Job drawing, mm, ordinate dimensions from the low corner. One solid piece. A direction names the side the tool comes from. Round coordinates to 2 decimals unless told otherwise and drop trailing zeros. Write each loop counter-clockwise with the first axis right and the second up, starting at its lowest first coordinate (ties: lowest second). Pieces come first, ordered by that corner, then holes.
1) Pull direction Z, two halves, no side cores. Call the marked faces 5, 6, 7 and 8: +Z half, -Z half, draft (parallel to the pull), parting line (faces both ways), or undercut.
2) Saw through at B-B on y = 34.5. Write the cut outline in (x, z), and give its area (3 significant figures).
3) Flat gauge pins, fed straight in: pin 1 (10 mm diameter, centred on x = 7, z = 17.5, fed in from -Y); pin 2 (3.5 mm diameter, centred on y = 23.5, z = 23.5, fed in from +X); pin 3 (0.6 mm diameter, centred on x = 30.5, y = 11, fed in from +Z); pin 4 (2.5 mm diameter, centred on x = 15, z = 15, fed in from +Y). Where does each tip first touch, or does it go through?
4) Saw through at D-D on y = 20.5. Write the cut outline in (x, z).
5) Which spindle directions (+Z, -Z, +X, -X, +Y, -Y) get a long thin tool onto all of the face, cutting with end or side? Do the marked faces 1, 2, 3 and 4. Say none if no direction does.
6) Drill centre lines: L1, parallel to Y at x = 27.5, z = 15; L2, parallel to Z at x = 4, y = 31; L3, parallel to X at y = 36, z = 6.5. Where is each one in solid material? Low to high.
7) Saw through at A-A on z = 15. Write the cut outline in (x, y), and give its area (3 significant figures).
8) Saw through at C-C on x = 15. Write the cut outline in (y, z), and give its area (3 significant figures).
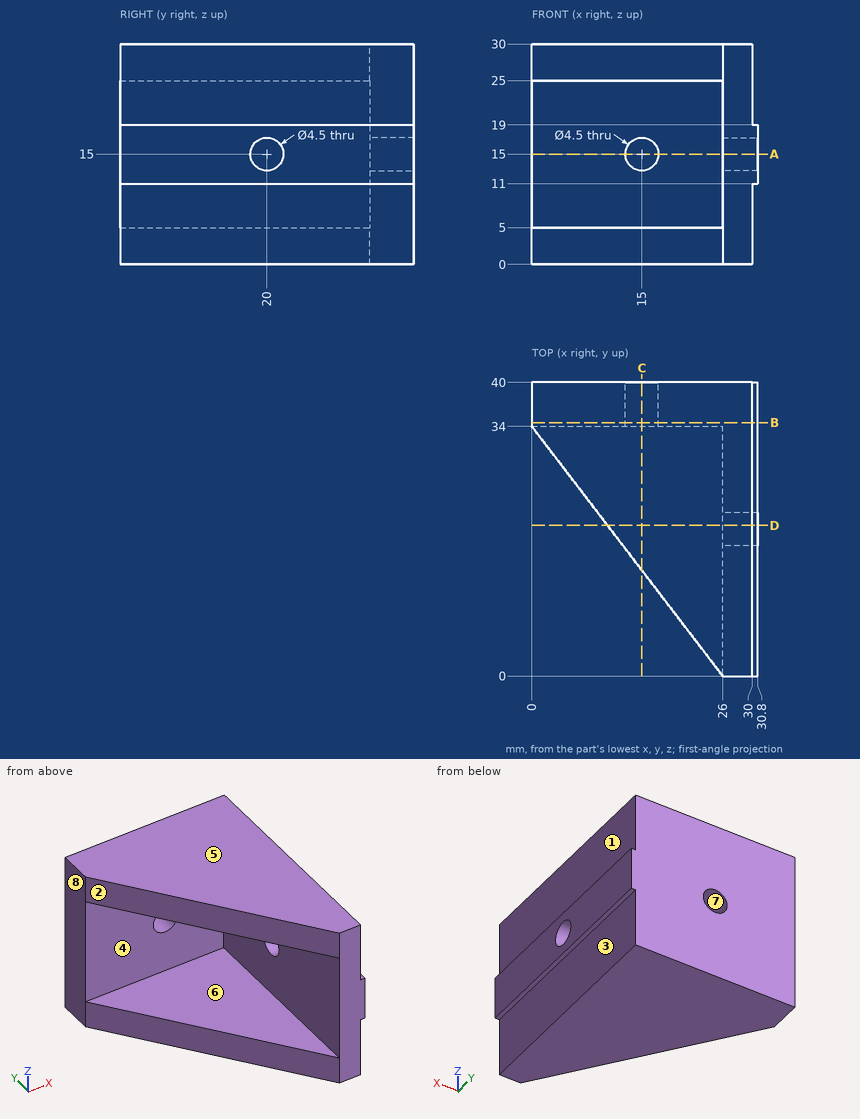
Completed:
1. face 5: +Z half
1. face 6: undercut
1. face 7: undercut
1. face 8: draft
2. outline: (0, 0) - (30, 0) - (30, 11) - (30.8, 11) - (30.8, 19) - (30, 19) - (30, 30) - (0, 30) - close; hole circle Ø4.5 at (15, 15)
2. area: 890 mm2
3. pin 1: stops at y = 34
3. pin 2: stops at x = 30
3. pin 3: stops at z = 19
3. pin 4: passes through
4. outline: (10.32, 0) - (30, 0) - (30, 11) - (30.8, 11) - (30.8, 12.81) - (26, 12.81) - (26, 5) - (10.32, 5) - close; (10.32, 25) - (26, 25) - (26, 17.19) - (30.8, 17.19) - (30.8, 19) - (30, 19) - (30, 30) - (10.32, 30) - close
5. face 1: +Z, +X, +Y, -Y
5. face 2: +Z, -Z, -X, -Y
5. face 3: -Z, +X, +Y, -Y
5. face 4: -X, -Y
6. L1: y = 0 to 17.75, 22.25 to 40
6. L2: z = 0 to 5, 25 to 30
6. L3: x = 0 to 30
7. outline: (0, 34) - (12.75, 34) - (12.75, 40) - (0, 40) - close; (17.25, 34) - (26, 34) - (26, 22.25) - (30.8, 22.25) - (30.8, 40) - (17.25, 40) - close; (26, 0) - (30.8, 0) - (30.8, 17.75) - (26, 17.75) - close
7. area: 299 mm2
8. outline: (14.38, 0) - (40, 0) - (40, 12.75) - (34, 12.75) - (34, 5) - (14.38, 5) - close; (14.38, 25) - (34, 25) - (34, 17.25) - (40, 17.25) - (40, 30) - (14.38, 30) - close
8. area: 349 mm2
